Design review of the part built by this model. Coordinates are the model's own, in mm. Face numbers are marked on the shaded views. A direction names the side the tool comes from. Give positions to 0.01 mm unless a question says otherwise; leave off trailing zeros. Loops run counter-clockwise (first coordinate to the right, second up) from the corner with the lowest first, then second, coordinate; pieces in that order, holes last. Notation, with made-up numbers: M 60.5,58 L 64.5,58 A27 cw 64.5,87 Z; hole C -3,85.5 d10. An arc over 180 degrees is marked long. Use a Markdown table: item, result. Add a question column.
(1) Add section C-C, the plane y = 205.5. Give the boundary of the cut face in (x, z), then the cut area to 3 significant figures.
(2) Add section B-B, the plane x = -12.5. Give the boundary of the cut face in (y, z), then the cut area to 3 significant figures.
(3) For the marked faces 1 and 2, list the 3-axis set-ups (+Z, -Z, +X, -X, +Y, -Y) from which the entire face can be reached by the end or side of a thin tool; tool diameter is ignored.
(4) For probe 1 along X at (y, z) = (223.5, 13); probe 2 along X at (y, z) = (19.5, 23.5), list the stretches that pass through material, from the lowest coordinate up.
(5) Add section A-A, the plane z = 2. Give the boundary of the cut face in (x, y).
(6) Draft analysis for pull direction Z (two halves, no side actions). For the marked faces 3, 4 and 5, state which applies: pulls with the +Z half, pulls with the -Z half, needs draft (parallel to the pull), parting line crosses it, or undercut.
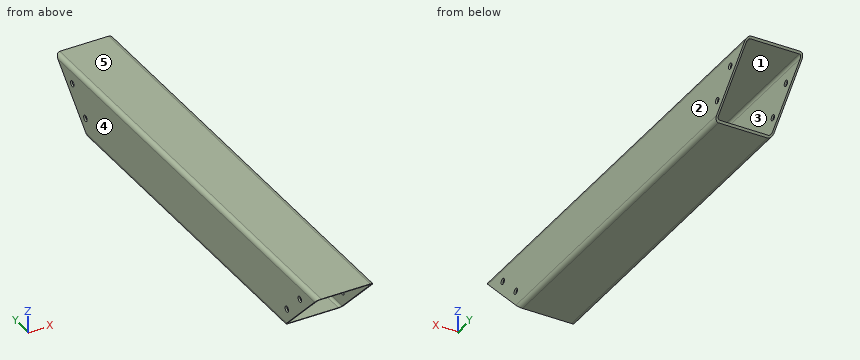
```python
from build123d import *

# Parameters (mm, degrees)
STRUCTURAL_MEMBER1_DEPTH = 425
CUT_EXTRUDE1_DEPTH       = 430.163657012
M5_CLEARANCE_HOLE1_D     = 5.5


with BuildPart() as part:
    # Sketch16 → Structural Member1 (new body)
    with BuildSketch(Plane.ZX):
        with BuildLine():
            Line((-26.67, 22.70125), (-26.67, -22.70125))
            ThreePointArc((-26.67, -22.70125), (-25.507580038, -25.507580038), (-22.70125, -26.67))
            Line((-22.70125, -26.67), (22.70125, -26.67))
            ThreePointArc((22.70125, -26.67), (25.507580038, -25.507580038), (26.67, -22.70125))
            Line((26.67, -22.70125), (26.67, 22.70125))
            ThreePointArc((26.67, 22.70125), (25.507580038, 25.507580038), (22.70125, 26.67))
            Line((22.70125, 26.67), (-22.70125, 26.67))
            ThreePointArc((-22.70125, 26.67), (-25.507580038, 25.507580038), (-26.67, 22.70125))
        make_face()
        with BuildLine():
            Line((-25.019, 22.70125), (-25.019, -22.70125))
            ThreePointArc((-25.019, -22.70125), (-24.340146742, -24.340146742), (-22.70125, -25.019))
            Line((-22.70125, -25.019), (22.70125, -25.019))
            ThreePointArc((22.70125, -25.019), (24.340146742, -24.340146742), (25.019, -22.70125))
            Line((25.019, -22.70125), (25.019, 22.70125))
            ThreePointArc((25.019, 22.70125), (24.340146742, 24.340146742), (22.70125, 25.019))
            Line((22.70125, 25.019), (-22.70125, 25.019))
            ThreePointArc((-22.70125, 25.019), (-24.340146742, 24.340146742), (-25.019, 22.70125))
        make_face(mode=Mode.SUBTRACT)
    extrude(amount=STRUCTURAL_MEMBER1_DEPTH)

    # Sketch12 → Cut-Extrude1 (cut, through all)
    with BuildSketch(Plane(origin=(26.67, 0, 0), x_dir=(0, 0, -1), z_dir=(1, 0, 0))):
        Polygon((-26.67, 425), (26.67, 371.66), (26.67, 425), align=None)
        Polygon((26.67, 0), (-26.67, 0), (26.67, 53.34), align=None)
    extrude(amount=-CUT_EXTRUDE1_DEPTH, mode=Mode.SUBTRACT)

    # M5 Clearance Hole1 (through all)
    with Locations(Plane(origin=(26.67, 0, 0), x_dir=(0, 0, -1), z_dir=(1, 0, 0))):
        with Locations((-12.02081528, 397.622893219), (9.192388155, 376.409689783), (-12.02081528, 28.084213562), (9.192388155, 49.297416998)):
            Hole(M5_CLEARANCE_HOLE1_D / 2)


solid = part.part
```
Established:
| question | item | result |
|---|---|---|
| 1 | outline | M -26.67,-22.7 A3.97 ccw -22.7,-26.67 L 22.7,-26.67 A3.97 ccw 26.67,-22.7 L 26.67,22.7 A3.97 ccw 22.7,26.67 L -22.7,26.67 A3.97 ccw -26.67,22.7 Z; hole M -25.02,-22.7 A2.32 ccw -22.7,-25.02 L 22.7,-25.02 A2.32 ccw 25.02,-22.7 L 25.02,22.7 A2.32 ccw 22.7,25.02 L -22.7,25.02 A2.32 ccw -25.02,22.7 Z |
| 1 | area | 332 mm^2 |
| 2 | outline | M 0,26.67 L 1.65,25.02 L 423.35,25.02 L 425,26.67 Z; M 51.69,-25.02 L 53.34,-26.67 L 371.66,-26.67 L 373.31,-25.02 Z |
| 2 | area | 1,230 mm^2 |
| 3 | face 1 | +Y, -Y |
| 3 | face 2 | +Z, -Z, +X, +Y, -Y |
| 4 | probe 1 | -26.67 to -25.02, 25.02 to 26.67 |
| 4 | probe 2 | -26.59 to -24.88, 24.88 to 26.59 |
| 5 | outline | M -26.67,24.67 L -25.02,24.67 L -25.02,400.33 L -26.67,400.33 Z; M 25.02,24.67 L 26.67,24.67 L 26.67,400.33 L 25.02,400.33 Z |
| 6 | face 3 | undercut |
| 6 | face 4 | needs draft |
| 6 | face 5 | pulls with the +Z half |
